Verification items for the finished model (mm, model axes). Face numbers are marked on the shaded views. A direction names the side the tool comes from. Coordinates: 2 decimals unless noted, no trailing zeros. Answer as CSV lines item,"result". Start each with the question number.
1. Gauge pin test, flat ends, axial feed: P1, Ø4, axis at x = 0, z = 12, coming from the -Y side (3 decimals); P2, Ø5, axis at y = -26, z = -17.5, coming from the +X side; P3, Ø2, axis at x = 0, z = 19, coming from the +Y side. Record the tip position at first contact, or that the pin passes through.
2. Release check for a two-part mould opening along X. For the marked faces 1, 2 and 3 record: pulls with the +X half, pulls with the -X half, needs draft (parallel to the pull), parting line crosses it, or undercut.
3. Material ranges on line 1 (X direction, y = -20.35, z = 0); line 2 (Z direction, x = -6, y = -26.2); line 3 (X direction, y = -24.5, z = 6), recorded low to high. Write a range as [from, to].
4. Cross-section at A-A (y = -26.5). State how many separate pieces and enclosed holes the cut face has, plus the area to 3 significant figures.
5. Set-up check for the marked faces 4, 5 and 6: record each of +Z, -Z, +X, -X, +Y, -Y from which the full face is reachable in a straight line by a thin tool's end or side.
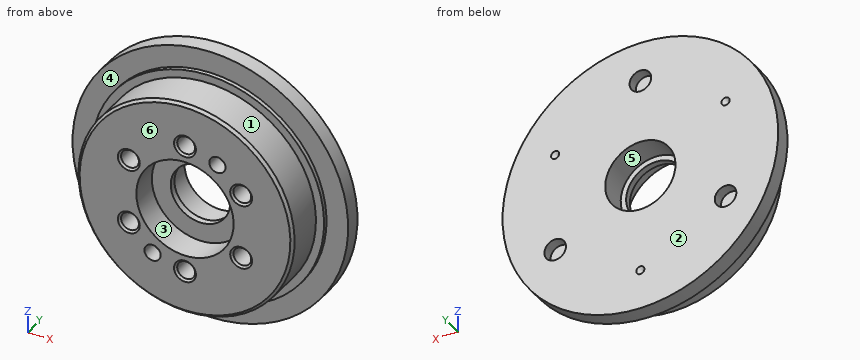
```python
from build123d import *

# Parameters (mm, degrees)
SKETCH_1_W                  = 25.5
SKETCH_1_H                  = 3
SKETCH_2_R                  = 21.5
EXTRUDE_1_DEPTH             = 0.8
SKETCH_3_R                  = 20
EXTRUDE_2_DEPTH             = 7.4
HOLE_WIZARD_3_0_3_1_D       = 3
HOLE_WIZARD_3_0_3_1_DEPTH   = 3
HOLE_WIZARD_3_3_3_3_1_D     = 3.3
HOLE_WIZARD_3_3_3_3_1_DEPTH = 8
HOLE_WIZARD_3_3_3_3_1_TIP   = 0.991420021
HOLE_WIZARD_4_0_4_1_D       = 4
HOLE_WIZARD_4_0_4_1_DEPTH   = 2
CHAMFER_1_SIZE              = 0.375
CHAMFER_2_SIZE              = 0.5


with BuildPart() as part:
    # 草图1 → 旋转1 (revolve)
    with BuildSketch(Plane.XY, mode=Mode.PRIVATE) as revolve_1_sk:
        with Locations((12.75, -18.3)):
            Rectangle(SKETCH_1_W, SKETCH_1_H)
    revolve(revolve_1_sk.sketch.rotate(Axis((0, -16.8, 0), (0, -1, 0)), 270), axis=Axis((0, -16.8, 0), (0, -1, 0)))

    # 草图2 → 凸台-拉伸1 (add)
    with BuildSketch(Plane.XZ.offset(19.8)):
        with Locations(Location((0, 0, 0), (0, 0, 90))):
            Circle(SKETCH_2_R)
    extrude(amount=EXTRUDE_1_DEPTH)

    # 草图3 → 凸台-拉伸2 (add)
    with BuildSketch(Plane.XZ.offset(20.6)):
        with Locations(Location((0, 0, 0), (0, 0, 270))):
            Circle(SKETCH_3_R)
    extrude(amount=EXTRUDE_2_DEPTH)

    # 草图4 → 切除-旋转1 (revolve, cut)
    with BuildSketch(Plane.XY.offset(9.1), mode=Mode.PRIVATE) as cut_revolve_1_sk:
        Polygon((-15.010946194, -16.8), (-15.761662349, -16.8), (-15.761662349, -17.251075774), align=None)
    revolve(cut_revolve_1_sk.sketch.rotate(Axis((-15.761662349, -16.8, 9.1), (0, -1, 0)), 90), axis=Axis((-15.761662349, -16.8, 9.1), (0, -1, 0)), mode=Mode.SUBTRACT)

    # 草图5 → 切除-旋转2 (revolve, cut)
    with BuildSketch(Plane.XY.offset(9.1), mode=Mode.PRIVATE) as cut_revolve_2_sk:
        Polygon((16.512378504, -16.8), (15.761662349, -16.8), (15.761662349, -17.251075774), align=None)
    revolve(cut_revolve_2_sk.sketch.rotate(Axis((15.761662349, -16.8, 9.1), (0, -1, 0)), 90), axis=Axis((15.761662349, -16.8, 9.1), (0, -1, 0)), mode=Mode.SUBTRACT)

    # 草图6 → 切除-旋转3 (revolve, cut)
    with BuildSketch(Plane.XY.offset(-18.2), mode=Mode.PRIVATE) as cut_revolve_3_sk:
        Polygon((0.750716155, -16.8), (0, -16.8), (0, -17.251075774), align=None)
    revolve(cut_revolve_3_sk.sketch.rotate(Axis((0, -16.8, -18.2), (0, -1, 0)), 90), axis=Axis((0, -16.8, -18.2), (0, -1, 0)), mode=Mode.SUBTRACT)

    # 草图7 → 切除-旋转4 (revolve, cut)
    with BuildSketch(Plane(origin=(0, 0, 0), x_dir=(-1, 0, 0), z_dir=(0, 0, -1)), mode=Mode.PRIVATE) as cut_revolve_4_sk:
        Polygon((-9, -28), (0, -28), (0, -16.8), (-6.5, -16.8), (-6.5, -21.8), (-5.5, -21.8), (-5.5, -23), (-9, -23), align=None)
    revolve(cut_revolve_4_sk.sketch.rotate(Axis((0, -28, 0), (0, 1, 0)), 270), axis=Axis((0, -28, 0), (0, 1, 0)), mode=Mode.SUBTRACT)

    # Ø3.0 (3) 直径孔1
    with Locations(Plane(origin=(0, -28, 0), x_dir=(-1, 0, 0), z_dir=(0, -1, 0))):
        with Locations((6, 10.392304845), (-6, -10.392304845)):
            Hole(HOLE_WIZARD_3_0_3_1_D / 2, depth=HOLE_WIZARD_3_0_3_1_DEPTH)

    # Ø3.3 (3.3) 直径孔1
    with Locations(Plane(origin=(0, -28, 0), x_dir=(-1, 0, 0), z_dir=(0, -1, 0))):
        with Locations((10.392304845, -6), (0, -12), (-10.392304845, -6), (-10.392304845, 6), (0, 12), (10.392304845, 6)):
            Hole(HOLE_WIZARD_3_3_3_3_1_D / 2, depth=HOLE_WIZARD_3_3_3_3_1_DEPTH)
            with Locations((0, 0, -(HOLE_WIZARD_3_3_3_3_1_DEPTH + HOLE_WIZARD_3_3_3_3_1_TIP / 2))):  # 118° drill point
                Cone(0, HOLE_WIZARD_3_3_3_3_1_D / 2, HOLE_WIZARD_3_3_3_3_1_TIP, mode=Mode.SUBTRACT)

    # Ø4.0 (4) 直径孔1
    with Locations(Plane(origin=(0, -16.8, 0), x_dir=(1, 0, 0), z_dir=(0, 1, 0))):
        with Locations((15.761662349, 9.1), (0, -18.2), (-15.761662349, 9.1)):
            Hole(HOLE_WIZARD_4_0_4_1_D / 2, depth=HOLE_WIZARD_4_0_4_1_DEPTH)

    # 倒角1
    chamfer_1_edges = [part.edges().sort_by_distance(p)[0] for p in [
        (-12.042304845, -28, -6),
        (-1.65, -28, -12),
        (8.742304845, -28, -6),
        (8.742304845, -28, 6),
        (-1.65, -28, 12),
        (-12.042304845, -28, 6),
    ]]
    chamfer(chamfer_1_edges, length=CHAMFER_1_SIZE)

    # 倒角2
    chamfer_2_edges = [part.edges().sort_by_distance(p)[0] for p in [
        (0, -28, 20),
    ]]
    chamfer(chamfer_2_edges, length=CHAMFER_2_SIZE)


solid = part.part
```
Values follow:
1,P1,"stops at y = -27.975"
1,P2,"stops at x = 13.23"
1,P3,"stops at y = -18.8"
2,face 1,"parting line crosses it"
2,face 2,"needs draft"
2,face 3,"undercut"
3,line 1,"x = [-21.5, -6.5], [6.5, 21.5]"
3,line 2,"z = [-19.08, -11.89], [-8.89, -6.71], [6.71, 19.08]"
3,line 3,"x = [-19.08, -12.04], [-8.74, -6.71], [6.71, 8.74], [12.04, 19.08]"
4,separate pieces,"1"
4,enclosed holes,"9"
4,area,"937 mm²"
5,face 4,"-Y"
5,face 5,"+Y"
5,face 6,"+Z, -Z, +X, -X, -Y"
